Answer from the drawing. Dimensions are ordinates in mm from the lowest x, y and z of the part. A direction names the side the tool comes from. Coordinates: 2 decimals unless noted, no trailing zeros. Write each loop counter-clockwise with the first axis right and the second up, starting at its lowest first coordinate (ties: lowest second). Pieces come first, ordered by that corner, then holes. Notation, with made-up numbers: (78, 28.25) - (97, 28.25) arc R5 ccw to (97, 33.25) - close; hole circle Ø11 at (84, 16.5). An arc over 180 degrees is marked (long way). Use a Markdown table: item, result.
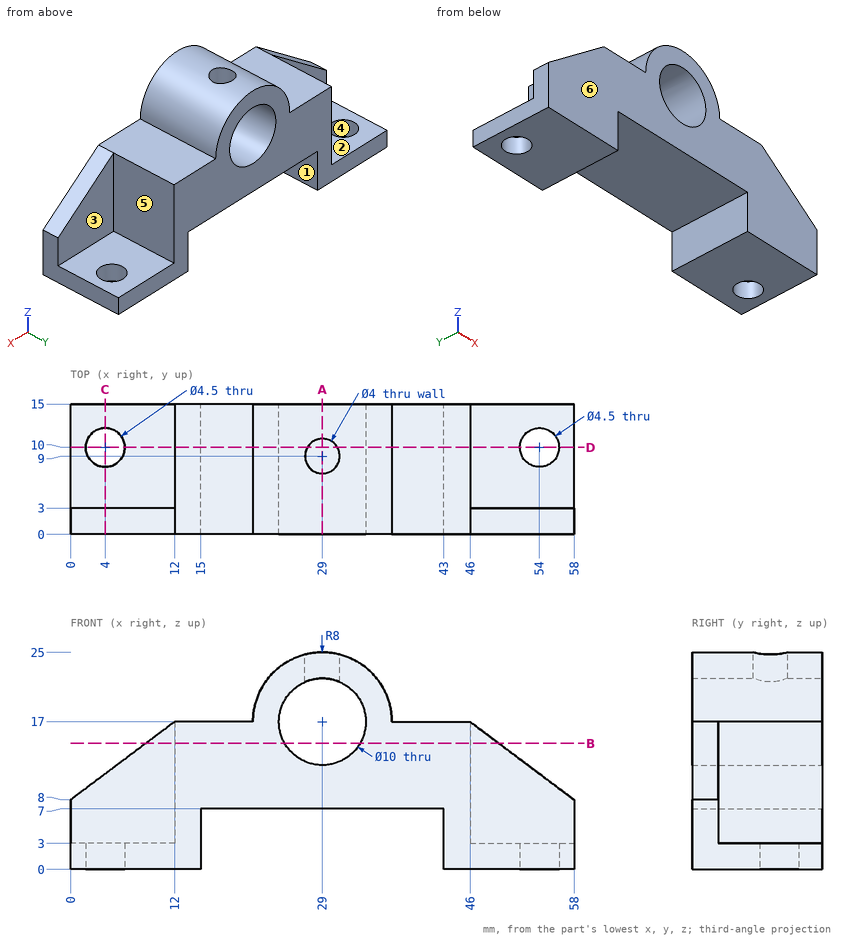
(1) A cutting plane is placed at B-B, the plane z = 14.5. Write down the section's boundary in (x, y), and give its area (3 significant figures).
Report:
| item | result |
|---|---|
| outline | (8.67, 0) - (24.67, 0) - (24.67, 15) - (12, 15) - (12, 3) - (8.67, 3) - close; (33.33, 0) - (49.33, 0) - (49.33, 3) - (46, 3) - (46, 15) - (33.33, 15) - close |
| area | 400 mm² |
(2) Each of these flat-tipped pins is pushed along its axis until it touches: P1, Ø3, axis at y = 7.5, z = 13, coming from the +X side; P2, Ø3.5, axis at x = 54, y = 10, coming from the +Z side; P3, Ø1, axis at x = 25.5, y = 7.5, coming from the -Z side; P4, Ø6, axis at x = 5, z = 11, coming from the +Y side. Where does it stop, or does it pass through?
Report:
| item | result |
|---|---|
| P1 | stops at x = 46 |
| P2 | passes through |
| P3 | stops at z = 7 |
| P4 | stops at y = 3 |
(3) A cutting plane is placed at A-A, the plane x = 29. Write down the section's boundary in (y, z), and give its area (3 significant figures).
Report:
| item | result |
|---|---|
| outline | (0, 7) - (15, 7) - (15, 12) - (0, 12) - close; (0, 22) - (7, 22) - (7, 25) - (0, 25) - close; (11, 22) - (15, 22) - (15, 25) - (11, 25) - close |
| area | 108 mm² |
(4) The mould has two halves that part along Y. Classify the marked faces 4, 5 and 6: pulls with the +Y half, pulls with the -Y half, needs draft (parallel to the pull), parting line crosses it, or undercut.
Report:
| item | result |
|---|---|
| face 4 | undercut |
| face 5 | needs draft |
| face 6 | pulls with the -Y half |
(5) Straight lines are drawn through the part: L1, parallel to Z at x = 29, y = 11.75; L2, parallel to Y at x = 4, z = 2.05; L3, parallel to Z at x = 39, y = 8.5. For each, find the intervals that lie inside material, in ascending order.
Report:
| item | result |
|---|---|
| L1 | z = 7 to 12, 22 to 25 |
| L2 | y = 0 to 7.75, 12.25 to 15 |
| L3 | z = 7 to 17 |
(6) A cutting plane is placed at C-C, the plane x = 4. Write down the section's boundary in (y, z).
Report:
| item | result |
|---|---|
| outline | (0, 0) - (7.75, 0) - (7.75, 3) - (3, 3) - (3, 11) - (0, 11) - close; (12.25, 0) - (15, 0) - (15, 3) - (12.25, 3) - close |
(7) For the marked faces 1, 2 and 3, determine the directions among +Z, -Z, +X, -X, +Y, -Y from which every point of the face is accessible in a straight line to the end or side of a thin tool.
Report:
| item | result |
|---|---|
| face 1 | -Z, +Y, -Y |
| face 2 | +Z, -X, +Y |
| face 3 | +Z, +X, +Y |
(8) A cutting plane is placed at D-D, the plane y = 10. Write down the section's boundary in (x, z), and give its area (3 significant figures).
Report:
| item | result |
|---|---|
| outline | (0, 0) - (1.75, 0) - (1.75, 3) - (0, 3) - close; (6.25, 0) - (15, 0) - (15, 7) - (43, 7) - (43, 0) - (51.75, 0) - (51.75, 3) - (46, 3) - (46, 17) - (37, 17) arc R8 ccw to (30.73, 24.81) - (30.73, 21.69) arc R5 cw (long way) to (27.27, 21.69) - (27.27, 24.81) arc R8 ccw to (21, 17) - (12, 17) - (12, 3) - (6.25, 3) - close; (56.25, 0) - (58, 0) - (58, 3) - (56.25, 3) - close |
| area | 438 mm² |
